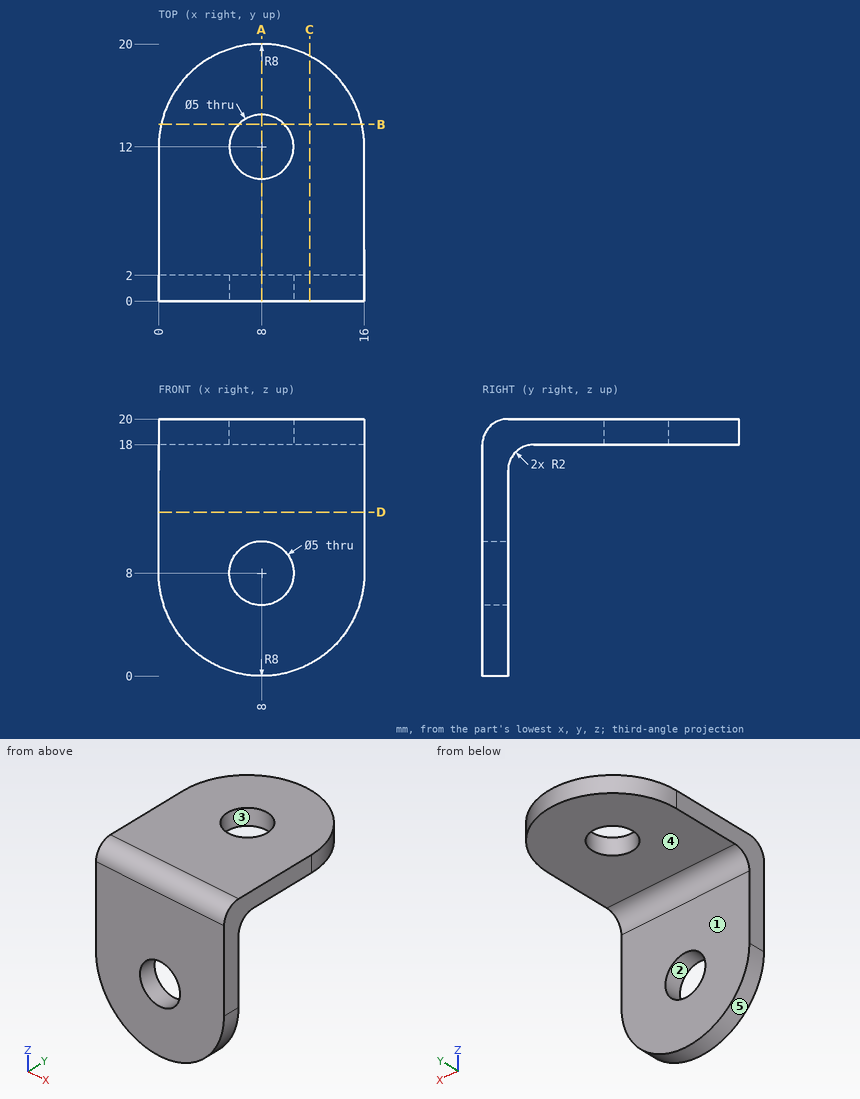
Check sheet for the drawn part. Datum: minimum x, y, z corner. Units: mm. A direction names the side the tool comes from. Round coordinates to 2 decimals unless told otherwise and drop trailing zeros. Order: outer loops, then holes, each group sorted by start corner. A loop starts at its lowest first (then second) coordinate and runs counter-clockwise, first axis right, second up. Notation, with made-up numbers: (24, -36.75) -> (33, -36.75) arc R28 cw to (33, -6.75) -> close; hole circle Ø5 at (15, 83.5). An arc over 180 degrees is marked (long way). Use CSV: the item, a comma, the result in double quotes.
(1) Draft check along Y on the marked faces 1, 2 and 3. Enter one of: pulls with the +Y half, pulls with the -Y half, needs draft (parallel to the pull), parting line crosses it, or undercut.
Worked out:
face 1,"pulls with the +Y half"
face 2,"needs draft"
face 3,"undercut"
(2) Cross-section at D-D (z = 12.75). Record the boundary of the cut face in (x, y), and give its area (3 significant figures).
Worked out:
outline,"(0, 0) -> (16, 0) -> (16, 2) -> (0, 2) -> close"
area,"32.0 mm²"
(3) Cross-section at B-B (y = 13.75). Record the boundary of the cut face in (x, z).
Worked out:
outline,"(0.19, 18) -> (6.21, 18) -> (6.21, 20) -> (0.19, 20) -> close; (9.79, 18) -> (15.81, 18) -> (15.81, 20) -> (9.79, 20) -> close"
(4) Depth check by flat-ended pin: pin 1 (8 mm diameter, centred on x = 9.5, y = 10.5, fed in from -Z); pin 2 (1.5 mm diameter, centred on y = 3, z = 16, fed in from -X); pin 3 (6 mm diameter, centred on x = 8, z = 8, fed in from +Y); pin 4 (6 mm diameter, centred on y = 15.5, z = 16, fed in from +X). Enter the tip coordinate at first touch or a pass-through.
Worked out:
pin 1,"z = 18"
pin 2,"through"
pin 3,"y = 2"
pin 4,"x = 15.9"
(5) Cross-section at A-A (x = 8). Record the boundary of the cut face in (y, z).
Worked out:
outline,"(0, 0) -> (2, 0) -> (2, 5.5) -> (0, 5.5) -> close; (0, 10.5) -> (2, 10.5) -> (2, 16) arc R2 cw to (4, 18) -> (9.5, 18) -> (9.5, 20) -> (2, 20) arc R2 ccw to (0, 18) -> close; (14.5, 18) -> (20, 18) -> (20, 20) -> (14.5, 20) -> close"
(6) Tool access check on the marked faces 4 and 5. Record the directions out of +Z, -Z, +X, -X, +Y, -Y that give a thin tool (end or side, any length) a straight path to the whole face; none if there is none.
Worked out:
face 4,"-Z, +X, -X, +Y"
face 5,"-Z, +Y, -Y"
(7) Cross-section at C-C (x = 11.75). Record the boundary of the cut face in (y, z).
Worked out:
outline,"(0, 0.93) -> (2, 0.93) -> (2, 16) arc R2 cw to (4, 18) -> (19.07, 18) -> (19.07, 20) -> (2, 20) arc R2 ccw to (0, 18) -> close"
(8) Material ranges on line 1 along X through (y, z) = (0.8, 8); line 2 along Y through (x, z) = (8, 18.65); line 3 along Y through (x, z) = (8, 19.2), recorded low to high. Write a range as from..to.
Worked out:
line 1,"0..5.5, 10.5..16"
line 2,"0.11..9.5, 14.5..20"
line 3,"0.4..9.5, 14.5..20"
